from build123d import *

# Parameters (mm, degrees)
SKETCH2_R = 2.5


with BuildPart() as part:
    # Sweep1: sweep along a path in Sketch1
    with BuildLine(Plane(origin=(0, 0, 0), x_dir=(0, 0, -1), z_dir=(1, 0, 0))) as sweep1_path:
        Line((0, 0), (-2, 0))
        ThreePointArc((-2, 0), (-4.828427125, 1.171572875), (-6, 4))
        Line((-6, 4), (-6, 30))
        ThreePointArc((-6, 30), (-3.071067812, 37.071067812), (4, 40))
        Line((4, 40), (19, 40))
        ThreePointArc((19, 40), (26.071067812, 37.071067812), (29, 30))
        Line((29, 30), (29, -20))
    # Sketch2 → Sweep1 (sweep)
    with BuildSketch(Plane.XY):
        Circle(SKETCH2_R)
    sweep(path=sweep1_path.line)


solid = part.part
Geometry check sheet. Reference: the model listing, model coordinates, mm. A direction names the side the tool comes from. Give positions to 0.01 mm unless a question says otherwise; leave off trailing zeros. Loops run counter-clockwise (first coordinate to the right, second up) from the corner with the lowest first, then second, coordinate; pieces in that order, holes last. Notation, with made-up numbers: M 88,10 L 124,10 A17 cw 124,14 Z; hole C -4,31.25 d11. An arc over 180 degrees is marked long. Answer as a JSON object with one key per item and string values. Group by question number.
Item 1: Gauge pin test, flat end, axial feed: pin 1 (2 mm diameter, centred on x = -2, y = 34, fed in from +Z). Record the tip position at first contact, or that the pin passes through.
Item 2: Sectioned sample at B-B on y = 8.5. Record the boundary of the cut face in (x, z).
Item 3: Sectioned sample at D-D on y = -12. Record the boundary of the cut face in (x, z).
Item 4: Sectioned sample at C-C on z = -9. Record the boundary of the cut face in (x, y), plus the area to 3 significant figures.
Item 5: Mould release check, pull along Z, two halves, no side actions. Record for faces 1 (the flat face through (0, 0, 0)), 2 (the flat face through (0, -20, -29)): pulls with the +Z half, pulls with the -Z half, needs draft (parallel to the pull), parting line crosses it, or undercut.
Item 6: Access from +Z, -Z, +X, -X, +Y, -Y to the whole of each face (thin tool, end or side, straight path). Record for faces 3 (the cylindrical face through (-0.33, 4.65, -26.52)), 4 (the cylindrical face through (-0.33, 17.18, 3.52)).
Item 7: Material ranges on L1, parallel to Z at x = 2.25, y = 18; L2, parallel to Z at x = 0.9, y = 9; L3, parallel to Z at x = 0.2, y = 40, recorded low to high.
Item 8: Sectioned sample at A-A on x = 0. Record the boundary of the cut face in (y, z), plus the area to 3 significant figures.
Findings below:
{
 "1": {"pin 1": "z = 7.72"},
 "2": {"outline": "C 0,-29 d5; C 0,6 d5"},
 "3": {"outline": "C 0,-29 d5"},
 "4": {"outline": "C 0,40 d5", "area": "19.6 mm2"},
 "5": {"face 1": "undercut", "face 2": "needs draft"},
 "6": {"face 3": "-Y", "face 4": "none"},
 "7": {"L1": "-30.09 to -27.91, 4.91 to 7.09", "L2": "-31.33 to -26.67, 3.67 to 8.33", "L3": "-26.49 to 3.49"},
 "8": {"outline": "M -20,-31.5 L 30,-31.5 A12.5 ccw 42.5,-19 L 42.5,-4 A12.5 ccw 30,8.5 L 4,8.5 A6.5 ccw -2.5,2 L -2.5,0 L 2.5,0 L 2.5,2 A1.5 cw 4,3.5 L 30,3.5 A7.5 cw 37.5,-4 L 37.5,-19 A7.5 cw 30,-26.5 L -20,-26.5 Z", "area": "653 mm2"}
}
